Geometry: final body of the model. Coordinates: model frame, mm. Give positions to 0.01 mm unless a question says otherwise; leave off trailing zeros. Write each loop counter-clockwise with the first axis right and the second up, starting at its lowest first coordinate (ties: lowest second). Pieces come first, ordered by that corner, then holes.
```python
from build123d import *

# Parameters (mm, degrees)
SKETCH1_W                     = 150
SKETCH1_H                     = 220
BOSS_EXTRUDE1_DEPTH           = 5
SKETCH2_R                     = 2.25
SKETCH2_R_2                   = 3
CUT_EXTRUDE2_DEPTH            = 10
SKETCH3_R                     = 5
CUT_EXTRUDE3_DEPTH            = 1
CUT_EXTRUDE3_DRAFT            = -60
CUT_EXTRUDE3_PROFILE_2_DEPTH  = 1
CUT_EXTRUDE3_PROFILE_2_DRAFT  = -60
CUT_EXTRUDE3_PROFILE_3_DEPTH  = 1
CUT_EXTRUDE3_PROFILE_3_DRAFT  = -60
CUT_EXTRUDE3_PROFILE_4_DEPTH  = 1
CUT_EXTRUDE3_PROFILE_4_DRAFT  = -60
CUT_EXTRUDE3_PROFILE_5_DEPTH  = 1
CUT_EXTRUDE3_PROFILE_5_DRAFT  = -60
CUT_EXTRUDE3_PROFILE_6_DEPTH  = 1
CUT_EXTRUDE3_PROFILE_6_DRAFT  = -60
CUT_EXTRUDE3_PROFILE_7_DEPTH  = 1
CUT_EXTRUDE3_PROFILE_7_DRAFT  = -60
CUT_EXTRUDE3_PROFILE_8_DEPTH  = 1
CUT_EXTRUDE3_PROFILE_8_DRAFT  = -60
CUT_EXTRUDE3_PROFILE_9_DEPTH  = 1
CUT_EXTRUDE3_PROFILE_9_DRAFT  = -60
CUT_EXTRUDE3_PROFILE_10_DEPTH = 1
CUT_EXTRUDE3_PROFILE_10_DRAFT = -60
CUT_EXTRUDE3_PROFILE_11_DEPTH = 1
CUT_EXTRUDE3_PROFILE_11_DRAFT = -60
CUT_EXTRUDE3_PROFILE_12_DEPTH = 1
CUT_EXTRUDE3_PROFILE_12_DRAFT = -60
FILLET1_R                     = 3


with BuildPart() as part:
    # Sketch1 → Boss-Extrude1 (new body)
    with BuildSketch(Plane(origin=(0, 0, 0), x_dir=(1, 0, 0), z_dir=(0, 1, 0))):
        with Locations((75, 110)):
            Rectangle(SKETCH1_W, SKETCH1_H)
    extrude(amount=-BOSS_EXTRUDE1_DEPTH)

    # Sketch2 → Cut-Extrude2 (cut)
    with BuildSketch(Plane(origin=(0, 0, 0), x_dir=(1, 0, 0), z_dir=(0, 1, 0))):
        with Locations(Location((11, 181, 0), (0, 0, 270))):
            Circle(SKETCH2_R)
        with Locations(Location((11, 157, 0), (0, 0, 270))):
            Circle(SKETCH2_R)
        with Locations(Location((29, 157, 0), (0, 0, 270))):
            Circle(SKETCH2_R)
        with Locations(Location((29, 181, 0), (0, 0, 270))):
            Circle(SKETCH2_R)
        with Locations(Location((11, 63, 0), (0, 0, 270))):
            Circle(SKETCH2_R)
        with Locations(Location((29, 63, 0), (0, 0, 270))):
            Circle(SKETCH2_R)
        with Locations(Location((11, 39, 0), (0, 0, 270))):
            Circle(SKETCH2_R)
        with Locations(Location((29, 39, 0), (0, 0, 270))):
            Circle(SKETCH2_R)
        with Locations(Location((119, 120, 0), (0, 0, 270))):
            Circle(SKETCH2_R_2)
        with Locations(Location((139, 120, 0), (0, 0, 270))):
            Circle(SKETCH2_R_2)
        with Locations(Location((119, 100, 0), (0, 0, 270))):
            Circle(SKETCH2_R_2)
        with Locations(Location((139, 100, 0), (0, 0, 270))):
            Circle(SKETCH2_R_2)
    extrude(amount=-CUT_EXTRUDE2_DEPTH, mode=Mode.SUBTRACT)


with BuildPart() as cut_extrude3_tool:
    # Sketch3 → Cut-Extrude3 (with draft: the straight prism first)
    with BuildSketch(Plane(origin=(0, 0, 0), x_dir=(1, 0, 0), z_dir=(0, 1, 0))):
        with Locations((11, 181)):
            Circle(SKETCH3_R)
    extrude(amount=-CUT_EXTRUDE3_DEPTH)
    # Cut-Extrude3: the draft: its side faces are tilted about the plane it starts from
    cut_extrude3_sides = [cut_extrude3_tool.faces().sort_by_distance(p)[0] for p in [
        (6, -0.5, -181),
    ]]
    draft(cut_extrude3_sides, Plane(origin=(0, 0, 0), x_dir=(1, 0, 0), z_dir=(0, 1, 0)), CUT_EXTRUDE3_DRAFT)


with BuildPart() as part_1:
    add(part.part)

    # Cut-Extrude3: cut by cut_extrude3_tool
    add(cut_extrude3_tool.part, mode=Mode.SUBTRACT)


with BuildPart() as cut_extrude3_profile_2_tool:
    # Sketch3 → Cut-Extrude3 profile 2 (with draft: the straight prism first)
    with BuildSketch(Plane(origin=(0, 0, 0), x_dir=(1, 0, 0), z_dir=(0, 1, 0))):
        with Locations((29, 181)):
            Circle(SKETCH3_R)
    extrude(amount=-CUT_EXTRUDE3_PROFILE_2_DEPTH)
    # Cut-Extrude3 profile 2: the draft: its side faces are tilted about the plane it starts from
    cut_extrude3_profile_2_sides = [cut_extrude3_profile_2_tool.faces().sort_by_distance(p)[0] for p in [
        (24, -0.5, -181),
    ]]
    draft(cut_extrude3_profile_2_sides, Plane(origin=(0, 0, 0), x_dir=(1, 0, 0), z_dir=(0, 1, 0)), CUT_EXTRUDE3_PROFILE_2_DRAFT)


with BuildPart() as part_2:
    add(part_1.part)

    # Cut-Extrude3 profile 2: cut by cut_extrude3_profile_2_tool
    add(cut_extrude3_profile_2_tool.part, mode=Mode.SUBTRACT)


with BuildPart() as cut_extrude3_profile_3_tool:
    # Sketch3 → Cut-Extrude3 profile 3 (with draft: the straight prism first)
    with BuildSketch(Plane(origin=(0, 0, 0), x_dir=(1, 0, 0), z_dir=(0, 1, 0))):
        with Locations((11, 157)):
            Circle(SKETCH3_R)
    extrude(amount=-CUT_EXTRUDE3_PROFILE_3_DEPTH)
    # Cut-Extrude3 profile 3: the draft: its side faces are tilted about the plane it starts from
    cut_extrude3_profile_3_sides = [cut_extrude3_profile_3_tool.faces().sort_by_distance(p)[0] for p in [
        (6, -0.5, -157),
    ]]
    draft(cut_extrude3_profile_3_sides, Plane(origin=(0, 0, 0), x_dir=(1, 0, 0), z_dir=(0, 1, 0)), CUT_EXTRUDE3_PROFILE_3_DRAFT)


with BuildPart() as part_3:
    add(part_2.part)

    # Cut-Extrude3 profile 3: cut by cut_extrude3_profile_3_tool
    add(cut_extrude3_profile_3_tool.part, mode=Mode.SUBTRACT)


with BuildPart() as cut_extrude3_profile_4_tool:
    # Sketch3 → Cut-Extrude3 profile 4 (with draft: the straight prism first)
    with BuildSketch(Plane(origin=(0, 0, 0), x_dir=(1, 0, 0), z_dir=(0, 1, 0))):
        with Locations((29, 157)):
            Circle(SKETCH3_R)
    extrude(amount=-CUT_EXTRUDE3_PROFILE_4_DEPTH)
    # Cut-Extrude3 profile 4: the draft: its side faces are tilted about the plane it starts from
    cut_extrude3_profile_4_sides = [cut_extrude3_profile_4_tool.faces().sort_by_distance(p)[0] for p in [
        (24, -0.5, -157),
    ]]
    draft(cut_extrude3_profile_4_sides, Plane(origin=(0, 0, 0), x_dir=(1, 0, 0), z_dir=(0, 1, 0)), CUT_EXTRUDE3_PROFILE_4_DRAFT)


with BuildPart() as part_4:
    add(part_3.part)

    # Cut-Extrude3 profile 4: cut by cut_extrude3_profile_4_tool
    add(cut_extrude3_profile_4_tool.part, mode=Mode.SUBTRACT)


with BuildPart() as cut_extrude3_profile_5_tool:
    # Sketch3 → Cut-Extrude3 profile 5 (with draft: the straight prism first)
    with BuildSketch(Plane(origin=(0, 0, 0), x_dir=(1, 0, 0), z_dir=(0, 1, 0))):
        with Locations((119, 120)):
            Circle(SKETCH3_R)
    extrude(amount=-CUT_EXTRUDE3_PROFILE_5_DEPTH)
    # Cut-Extrude3 profile 5: the draft: its side faces are tilted about the plane it starts from
    cut_extrude3_profile_5_sides = [cut_extrude3_profile_5_tool.faces().sort_by_distance(p)[0] for p in [
        (114, -0.5, -120),
    ]]
    draft(cut_extrude3_profile_5_sides, Plane(origin=(0, 0, 0), x_dir=(1, 0, 0), z_dir=(0, 1, 0)), CUT_EXTRUDE3_PROFILE_5_DRAFT)


with BuildPart() as part_5:
    add(part_4.part)

    # Cut-Extrude3 profile 5: cut by cut_extrude3_profile_5_tool
    add(cut_extrude3_profile_5_tool.part, mode=Mode.SUBTRACT)


with BuildPart() as cut_extrude3_profile_6_tool:
    # Sketch3 → Cut-Extrude3 profile 6 (with draft: the straight prism first)
    with BuildSketch(Plane(origin=(0, 0, 0), x_dir=(1, 0, 0), z_dir=(0, 1, 0))):
        with Locations((139, 120)):
            Circle(SKETCH3_R)
    extrude(amount=-CUT_EXTRUDE3_PROFILE_6_DEPTH)
    # Cut-Extrude3 profile 6: the draft: its side faces are tilted about the plane it starts from
    cut_extrude3_profile_6_sides = [cut_extrude3_profile_6_tool.faces().sort_by_distance(p)[0] for p in [
        (134, -0.5, -120),
    ]]
    draft(cut_extrude3_profile_6_sides, Plane(origin=(0, 0, 0), x_dir=(1, 0, 0), z_dir=(0, 1, 0)), CUT_EXTRUDE3_PROFILE_6_DRAFT)


with BuildPart() as part_6:
    add(part_5.part)

    # Cut-Extrude3 profile 6: cut by cut_extrude3_profile_6_tool
    add(cut_extrude3_profile_6_tool.part, mode=Mode.SUBTRACT)


with BuildPart() as cut_extrude3_profile_7_tool:
    # Sketch3 → Cut-Extrude3 profile 7 (with draft: the straight prism first)
    with BuildSketch(Plane(origin=(0, 0, 0), x_dir=(1, 0, 0), z_dir=(0, 1, 0))):
        with Locations((119, 100)):
            Circle(SKETCH3_R)
    extrude(amount=-CUT_EXTRUDE3_PROFILE_7_DEPTH)
    # Cut-Extrude3 profile 7: the draft: its side faces are tilted about the plane it starts from
    cut_extrude3_profile_7_sides = [cut_extrude3_profile_7_tool.faces().sort_by_distance(p)[0] for p in [
        (114, -0.5, -100),
    ]]
    draft(cut_extrude3_profile_7_sides, Plane(origin=(0, 0, 0), x_dir=(1, 0, 0), z_dir=(0, 1, 0)), CUT_EXTRUDE3_PROFILE_7_DRAFT)


with BuildPart() as part_7:
    add(part_6.part)

    # Cut-Extrude3 profile 7: cut by cut_extrude3_profile_7_tool
    add(cut_extrude3_profile_7_tool.part, mode=Mode.SUBTRACT)


with BuildPart() as cut_extrude3_profile_8_tool:
    # Sketch3 → Cut-Extrude3 profile 8 (with draft: the straight prism first)
    with BuildSketch(Plane(origin=(0, 0, 0), x_dir=(1, 0, 0), z_dir=(0, 1, 0))):
        with Locations((139, 100)):
            Circle(SKETCH3_R)
    extrude(amount=-CUT_EXTRUDE3_PROFILE_8_DEPTH)
    # Cut-Extrude3 profile 8: the draft: its side faces are tilted about the plane it starts from
    cut_extrude3_profile_8_sides = [cut_extrude3_profile_8_tool.faces().sort_by_distance(p)[0] for p in [
        (134, -0.5, -100),
    ]]
    draft(cut_extrude3_profile_8_sides, Plane(origin=(0, 0, 0), x_dir=(1, 0, 0), z_dir=(0, 1, 0)), CUT_EXTRUDE3_PROFILE_8_DRAFT)


with BuildPart() as part_8:
    add(part_7.part)

    # Cut-Extrude3 profile 8: cut by cut_extrude3_profile_8_tool
    add(cut_extrude3_profile_8_tool.part, mode=Mode.SUBTRACT)


with BuildPart() as cut_extrude3_profile_9_tool:
    # Sketch3 → Cut-Extrude3 profile 9 (with draft: the straight prism first)
    with BuildSketch(Plane(origin=(0, 0, 0), x_dir=(1, 0, 0), z_dir=(0, 1, 0))):
        with Locations((29, 63)):
            Circle(SKETCH3_R)
    extrude(amount=-CUT_EXTRUDE3_PROFILE_9_DEPTH)
    # Cut-Extrude3 profile 9: the draft: its side faces are tilted about the plane it starts from
    cut_extrude3_profile_9_sides = [cut_extrude3_profile_9_tool.faces().sort_by_distance(p)[0] for p in [
        (24, -0.5, -63),
    ]]
    draft(cut_extrude3_profile_9_sides, Plane(origin=(0, 0, 0), x_dir=(1, 0, 0), z_dir=(0, 1, 0)), CUT_EXTRUDE3_PROFILE_9_DRAFT)


with BuildPart() as part_9:
    add(part_8.part)

    # Cut-Extrude3 profile 9: cut by cut_extrude3_profile_9_tool
    add(cut_extrude3_profile_9_tool.part, mode=Mode.SUBTRACT)


with BuildPart() as cut_extrude3_profile_10_tool:
    # Sketch3 → Cut-Extrude3 profile 10 (with draft: the straight prism first)
    with BuildSketch(Plane(origin=(0, 0, 0), x_dir=(1, 0, 0), z_dir=(0, 1, 0))):
        with Locations((11, 63)):
            Circle(SKETCH3_R)
    extrude(amount=-CUT_EXTRUDE3_PROFILE_10_DEPTH)
    # Cut-Extrude3 profile 10: the draft: its side faces are tilted about the plane it starts from
    cut_extrude3_profile_10_sides = [cut_extrude3_profile_10_tool.faces().sort_by_distance(p)[0] for p in [
        (6, -0.5, -63),
    ]]
    draft(cut_extrude3_profile_10_sides, Plane(origin=(0, 0, 0), x_dir=(1, 0, 0), z_dir=(0, 1, 0)), CUT_EXTRUDE3_PROFILE_10_DRAFT)


with BuildPart() as part_10:
    add(part_9.part)

    # Cut-Extrude3 profile 10: cut by cut_extrude3_profile_10_tool
    add(cut_extrude3_profile_10_tool.part, mode=Mode.SUBTRACT)


with BuildPart() as cut_extrude3_profile_11_tool:
    # Sketch3 → Cut-Extrude3 profile 11 (with draft: the straight prism first)
    with BuildSketch(Plane(origin=(0, 0, 0), x_dir=(1, 0, 0), z_dir=(0, 1, 0))):
        with Locations((11, 39)):
            Circle(SKETCH3_R)
    extrude(amount=-CUT_EXTRUDE3_PROFILE_11_DEPTH)
    # Cut-Extrude3 profile 11: the draft: its side faces are tilted about the plane it starts from
    cut_extrude3_profile_11_sides = [cut_extrude3_profile_11_tool.faces().sort_by_distance(p)[0] for p in [
        (6, -0.5, -39),
    ]]
    draft(cut_extrude3_profile_11_sides, Plane(origin=(0, 0, 0), x_dir=(1, 0, 0), z_dir=(0, 1, 0)), CUT_EXTRUDE3_PROFILE_11_DRAFT)


with BuildPart() as part_11:
    add(part_10.part)

    # Cut-Extrude3 profile 11: cut by cut_extrude3_profile_11_tool
    add(cut_extrude3_profile_11_tool.part, mode=Mode.SUBTRACT)


with BuildPart() as cut_extrude3_profile_12_tool:
    # Sketch3 → Cut-Extrude3 profile 12 (with draft: the straight prism first)
    with BuildSketch(Plane(origin=(0, 0, 0), x_dir=(1, 0, 0), z_dir=(0, 1, 0))):
        with Locations((29, 39)):
            Circle(SKETCH3_R)
    extrude(amount=-CUT_EXTRUDE3_PROFILE_12_DEPTH)
    # Cut-Extrude3 profile 12: the draft: its side faces are tilted about the plane it starts from
    cut_extrude3_profile_12_sides = [cut_extrude3_profile_12_tool.faces().sort_by_distance(p)[0] for p in [
        (24, -0.5, -39),
    ]]
    draft(cut_extrude3_profile_12_sides, Plane(origin=(0, 0, 0), x_dir=(1, 0, 0), z_dir=(0, 1, 0)), CUT_EXTRUDE3_PROFILE_12_DRAFT)


with BuildPart() as part_12:
    add(part_11.part)

    # Cut-Extrude3 profile 12: cut by cut_extrude3_profile_12_tool
    add(cut_extrude3_profile_12_tool.part, mode=Mode.SUBTRACT)

    # Fillet1
    fillet1_edges = [part_12.edges().sort_by_distance(p)[0] for p in [
        (150, -2.5, -220),
        (150, -2.5, 0),
        (0, -2.5, 0),
        (0, -2.5, -220),
    ]]
    fillet(fillet1_edges, radius=FILLET1_R)


solid = part_12.part
```
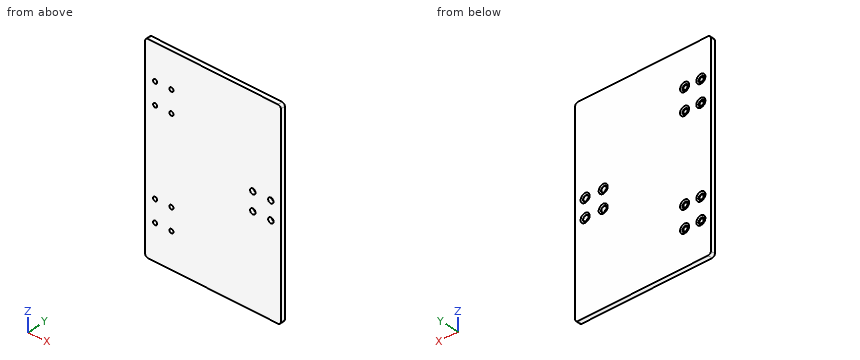
Item 1: Section B-B, the plane x = 119. Return the cut outline in (y, z).
Found:
outline: (-5, -220) - (0, -220) - (0, -125) - (-1, -123.27) - (-1, -123) - (-5, -123) - close; (-5, -117) - (-1, -117) - (-1, -116.73) - (0, -115) - (0, -105) - (-1, -103.27) - (-1, -103) - (-5, -103) - close; (-5, -97) - (-1, -97) - (-1, -96.73) - (0, -95) - (0, 0) - (-5, 0) - close
Item 2: Section C-C, the plane x = 11. State how many separate pieces and enclosed holes the cut face has, plus the area to 3 significant figures.
Found:
separate pieces: 5
enclosed holes: 0
area: 995 mm2
Item 3: Section A-A, the plane z = -100. Return the cut outline in (x, y).
Found:
outline: (0, -5) - (116, -5) - (116, -1) - (115.73, -1) - (114, 0) - (0, 0) - close; (122, -5) - (136, -5) - (136, -1) - (135.73, -1) - (134, 0) - (124, 0) - (122.27, -1) - (122, -1) - close; (142, -5) - (150, -5) - (150, 0) - (144, 0) - (142.27, -1) - (142, -1) - close
Item 4: Line query: L1, parallel to X at y = -4.1, z = -63; L2, parallel to Z at x = 139, y = -2.7; L3, parallel to X at y = -2, z = -62. Output: solid intervals per line, ascending.
Found:
L1: x = 0 to 8.75, 13.25 to 26.75, 31.25 to 150
L2: z = -220 to -123, -117 to -103, -97 to 0
L3: x = 0 to 8.98, 13.02 to 26.98, 31.02 to 150
Item 5: Pin query (flat end, axial travel): pin 1 Ø7 at (x, z) = (29, -63) entering from -Y; pin 2 Ø5 at (x, z) = (118.5, -119.5) entering from +Y; pin 3 Ø5 at (x, z) = (30, -156) entering from +Y; pin 4 Ø9.5 at (x, z) = (139, -100) entering from +Y. Return the tip coordinate at first contact, or that it passes through.
Found:
pin 1: stops at y = -5
pin 2: stops at y = -1
pin 3: stops at y = -0.63
pin 4: stops at y = -0.14
